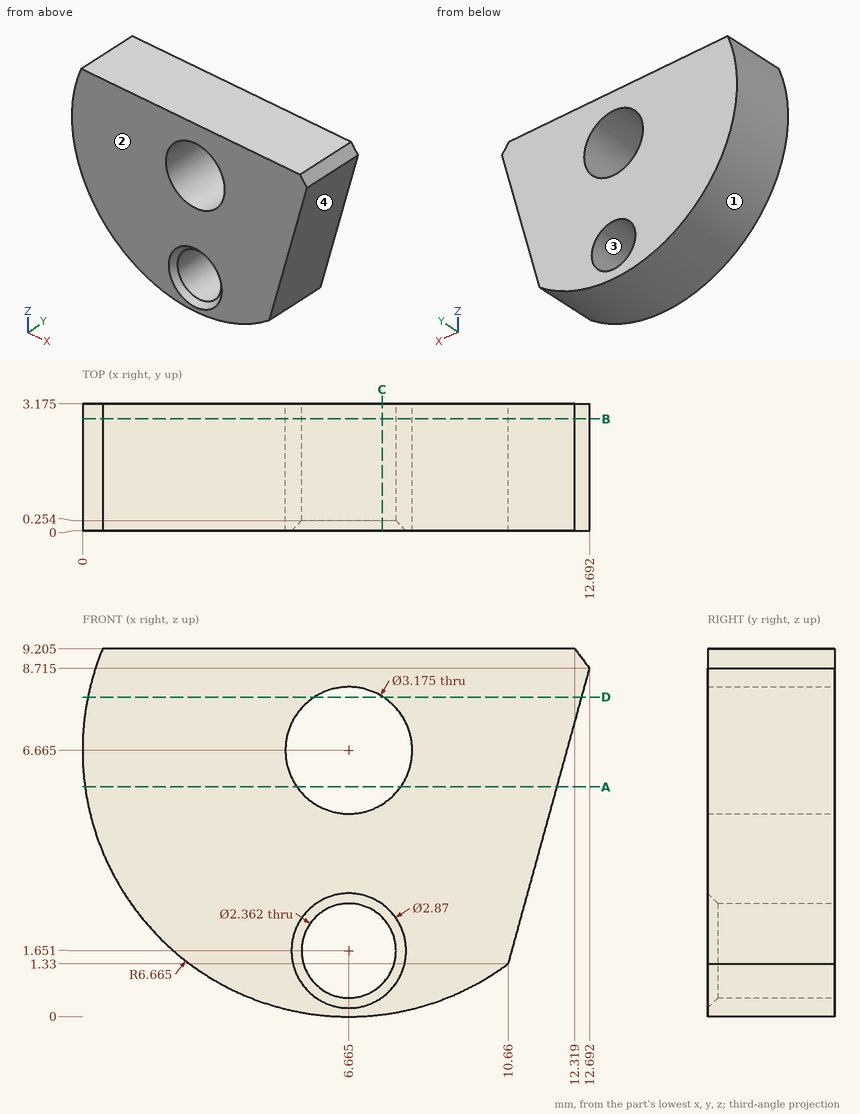
Job drawing, mm, ordinate dimensions from the low corner. One solid piece. Round coordinates to 2 decimals unless told otherwise and drop trailing zeros. Loops run counter-clockwise (first coordinate to the right, second up) from the corner with the lowest first, then second, coordinate; pieces in that order, holes last. Notation, with made-up numbers: M 23,-18 L 33,-18 A11 ccw 33,-3 Z; hole C 43.5,85 d1. An arc over 180 degrees is marked long. One line per question, with ' | ' between items. Start each with the question number.
Item 1: Wall check: line 1 (Z direction, x = 5.75, y = 1.6) (1 decimal); line 2 (X direction, y = 0.7, z = 7.75) (1 decimal); line 3 (Z direction, x = 8.5, y = 2.25) (1 decimal). Give the ranges that are in metal, low to high.
Item 2: Cut at B-B, the plane y = 2.8. Write the cut outline in (x, z) (1 decimal).
Item 3: Cut at D-D, the plane z = 8. Write the cut outline in (x, y) (1 decimal), plus the area to 3 significant figures.
Item 4: Cut at C-C, the plane x = 7.5. State how many separate pieces and enclosed holes the cut face has, plus the area to 3 significant figures.
Item 5: Two-plate mould, pull along X, no slides. Class the marked faces 1, 2, 3 and 4: pulls with the +X half, pulls with the -X half, needs draft (parallel to the pull), parting line crosses it, or undercut.
Item 6: Cut at A-A, the plane z = 5.75. Write the cut outline in (x, y) (1 decimal).
Responses:
1) line 1: z = 0.1 to 0.9, 2.4 to 5.4, 8 to 9.2 | line 2: x = 0.1 to 5.5, 7.8 to 12.4 | line 3: z = 0.3 to 9.2
2) outline: M 0.5,9.2 A6.7 ccw 10.7,1.3 L 12.7,8.7 L 12.3,9.2 Z; hole C 6.7,6.7 d3.2; hole C 6.7,1.7 d2.4
3) outline: M 0.1,0 L 5.8,0 L 5.8,3.2 L 0.1,3.2 Z; M 7.5,0 L 12.5,0 L 12.5,3.2 L 7.5,3.2 Z | area: 33.8 mm²
4) separate pieces: 3 | enclosed holes: 0 | area: 15.1 mm²
5) face 1: parting line crosses it | face 2: needs draft | face 3: undercut | face 4: pulls with the +X half
6) outline: M 0.1,0 L 5.4,0 L 5.4,3.2 L 0.1,3.2 Z; M 8,0 L 11.9,0 L 11.9,3.2 L 8,3.2 Z
